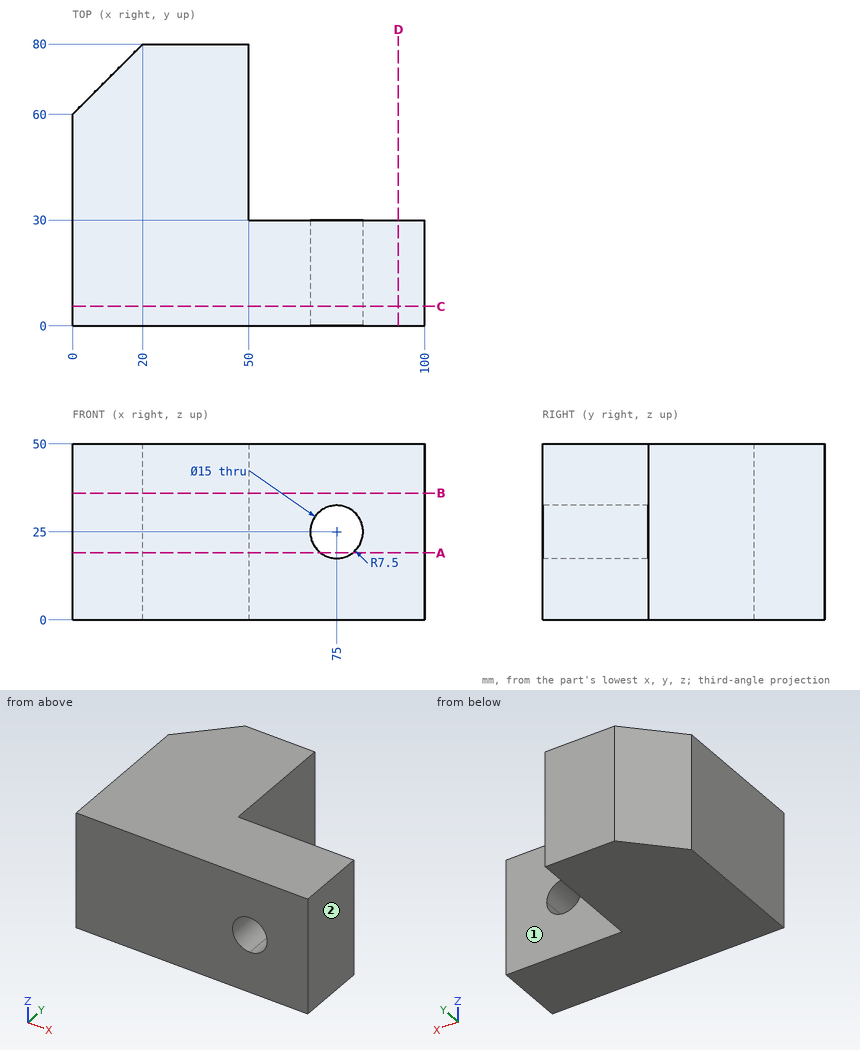
For this review, use the dimensioned drawing (mm, ordinates from the lowest corner) and the shaded views. A direction names the side the tool comes from. Coordinates: 2 decimals unless noted, no trailing zeros. Loops run counter-clockwise (first coordinate to the right, second up) from the corner with the lowest first, then second, coordinate; pieces in that order, holes last.
1. Insertion check: P1, Ø15, axis at x = 86, z = 34, coming from the +Y side; P2, Ø1, axis at x = 17, z = 14.5, coming from the +Y side; P3, Ø3, axis at y = 40, z = 44, coming from the +X side. Each pin has a flat end and moves straight along its axis. Give the tip position at first contact, or say it passes through.
2. Add section A-A, the plane z = 19. Give the boundary of the cut face in (x, y).
3. For line 1 (X direction, y = 19.25, z = 25); line 2 (Z direction, x = 75, y = 7); line 3 (Y direction, x = 88.5, z = 43), list the stretches that pass through material, from the lowest coordinate up.
4. For the marked faces 1 and 2, list the 3-axis set-ups (+Z, -Z, +X, -X, +Y, -Y) from which the entire face can be reached by the end or side of a thin tool; tool diameter is ignored.
5. Add section D-D, the plane x = 92.5. Give the boundary of the cut face in (y, z), then the cut area to 3 significant figures.
6. Add section C-C, the plane y = 5.5. Give the boundary of the cut face in (x, z).
7. Add section B-B, the plane z = 36. Give the boundary of the cut face in (x, y).
Result:
1. P1: stops at y = 30
1. P2: stops at y = 77.5
1. P3: stops at x = 50
2. outline: (0, 0) - (70.5, 0) - (70.5, 30) - (50, 30) - (50, 80) - (20, 80) - (0, 60) - close; (79.5, 0) - (100, 0) - (100, 30) - (79.5, 30) - close
3. line 1: x = 0 to 67.5, 82.5 to 100
3. line 2: z = 0 to 17.5, 32.5 to 50
3. line 3: y = 0 to 30
4. face 1: +Z, -Z, +X, +Y
4. face 2: +Z, -Z, +X, +Y, -Y
5. outline: (0, 0) - (30, 0) - (30, 50) - (0, 50) - close
5. area: 1,500 mm2
6. outline: (0, 0) - (100, 0) - (100, 50) - (0, 50) - close; hole circle Ø15 at (75, 25)
7. outline: (0, 0) - (100, 0) - (100, 30) - (50, 30) - (50, 80) - (20, 80) - (0, 60) - close
